Check sheet for the drawn part. Datum: minimum x, y, z corner. Units: mm. Round coordinates to 2 decimals unless told otherwise and drop trailing zeros. Order: outer loops, then holes, each group sorted by start corner. A loop starts at its lowest first (then second) coordinate and runs counter-clockwise, first axis right, second up.
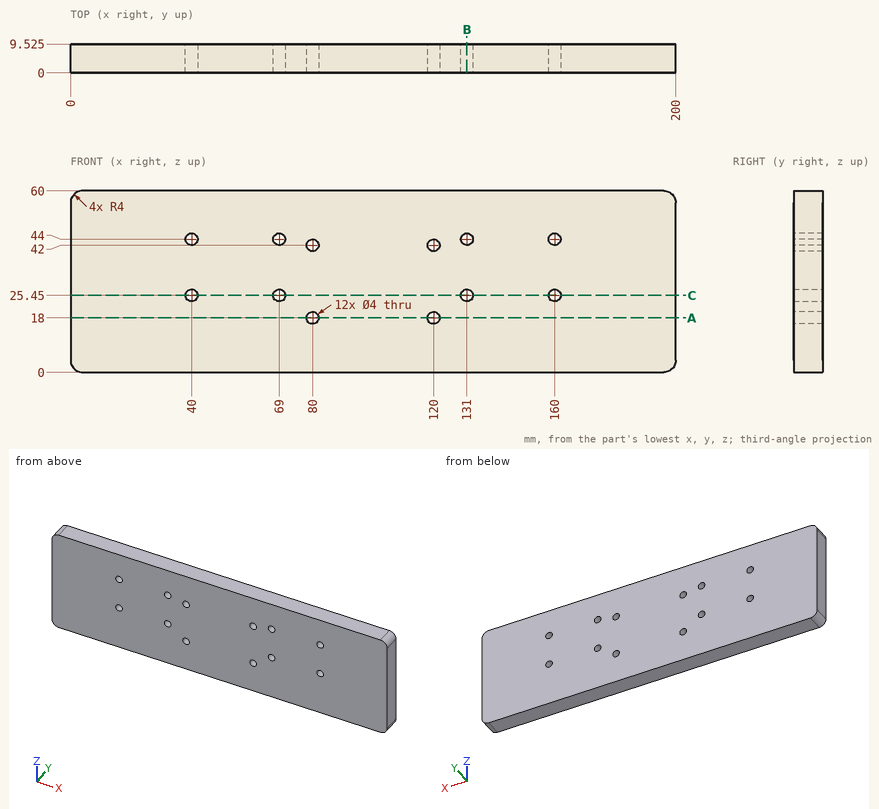
1) Sectioned sample at C-C on z = 25.45. Record the cut outline in (x, y) (3 decimals).
2) Sectioned sample at B-B on x = 131. Record the cut outline in (y, z) (3 decimals).
3) Gauge pin test, flat end, axial feed: pin 1 (3 mm diameter, centred on x = 160, z = 25.45, fed in from +Y). Record the tip position at first contact, or that the pin passes through.
4) Scan lines: line 1 (Z direction, x = 80, y = 4.25); line 2 (Z direction, x = 160, y = 4). Record each from-to range of solid material in increasing order.
5) Sectioned sample at A-A on z = 18. Record the cut outline in (x, y) (3 decimals), and give its area (3 significant figures).
Values found:
1. outline: (0, 0) - (38, 0) - (38, 9.525) - (0, 9.525) - close; (42, 0) - (67, 0) - (67, 9.525) - (42, 9.525) - close; (71, 0) - (129, 0) - (129, 9.525) - (71, 9.525) - close; (133, 0) - (158, 0) - (158, 9.525) - (133, 9.525) - close; (162, 0) - (200, 0) - (200, 9.525) - (162, 9.525) - close
2. outline: (0, 0) - (9.525, 0) - (9.525, 23.45) - (0, 23.45) - close; (0, 27.45) - (9.525, 27.45) - (9.525, 42) - (0, 42) - close; (0, 46) - (9.525, 46) - (9.525, 60) - (0, 60) - close
3. pin 1: passes through
4. line 1: z = 0 to 16, 20 to 40, 44 to 60
4. line 2: z = 0 to 23.45, 27.45 to 42, 46 to 60
5. outline: (0, 0) - (78, 0) - (78, 9.525) - (0, 9.525) - close; (82, 0) - (118, 0) - (118, 9.525) - (82, 9.525) - close; (122, 0) - (200, 0) - (200, 9.525) - (122, 9.525) - close
5. area: 1,830 mm2
